Part model, mm, in its own coordinate system. A direction names the side the tool comes from. Give positions to 0.01 mm unless a question says otherwise; leave off trailing zeros. Write each loop counter-clockwise with the first axis right and the second up, starting at its lowest first coordinate (ties: lowest second). Pieces come first, ordered by that corner, then holes. Notation, with made-up numbers: M 83,-6 L 132,-6 A28 cw 132,19 Z; hole C -35,-8.5 d3. An arc over 180 degrees is marked long. Use CSV: the item, a comma, the result in double quotes. Start each with the question number.
1. 3-axis set-ups, long thin cutter, end or side, ignore diameter. For faces 1 (the face through (11, -7.62, 1)), 2 (the face through (3, -4, 22.86)), 3 (the face through (3, -5.08, 37)), 4 (the face through (8, -5, 20.32)), 5 (the face through (5.08, -8, 13)): which of +Z, -Z, +X, -X, +Y, -Y reach the whole face in a straight line?
2. Drill centre lines: line 1 along Z through (x, y) = (2, -3.25); line 2 along X through (y, z) = (-3, 12); line 3 along Y through (x, z) = (5, 20.5). Where is each one in solid material? Low to high. Write a range as from..to.
3. Band-saw the part on A-A, the plane y = -3. List the corners of the cut face in (x, z), then the cut area to 3 significant figures.
4. Band-saw the part on D-D, the plane y = -6. List the corners of the cut face in (x, z), then the cut area to 3 significant figures.
5. Mould opens along Z. For faces 6 (the face through (3, -4, 27.94)), 7 (the face through (7.62, -11, 1)), 8 (the face through (3, -3, 45.72)) say: pulls with the +Z half, pulls with the -Z half, needs draft (parallel to the pull), parting line crosses it, or undercut.
6. Drop flat-ended pins along their axis: pin 1 Ø5 at (y, z) = (-2.5, 8) entering from +X; pin 2 Ø0.8 at (x, y) = (2, -4) entering from -Z; pin 3 Ø2.5 at (x, z) = (3.5, 25.5) entering from -Y; pin 4 Ø0.8 at (x, z) = (11.5, 2) entering from +Y. Give the stop position or say it passes through.
7. Band-saw the part on B-B, the plane x = 4. List the corners of the cut face in (y, z).
8. Band-saw the part on C-C, the plane z = 24. List the corners of the cut face in (x, y), then the cut area to 3 significant figures.
from build123d import *

# Parameters (mm, degrees)
F0_W     = 10.16
F0_H     = 10.16
F1_DEPTH = 5.08
F2_W     = 5.08
F2_H     = 5.08
F3_DEPTH = 2.54
F4_W     = 5.08
F4_H     = 5.08
F5_DEPTH = 40.64
F6_W     = 5.08
F6_H     = 5.08
F7_DEPTH = 25.4
F8_W     = 5.08
F8_H     = 10.16
F9_DEPTH = 15.24


with BuildPart() as f1:
    # F0 (on Top) → F1 (new body)
    with BuildSketch(Plane.XY):
        with Locations((5.08, -5.08)):
            Rectangle(F0_W, F0_H)
    extrude(amount=F1_DEPTH)

    # F2 (on face) → F3 (join)
    with BuildSketch(Plane(origin=(0, 0, 0), x_dir=(1, 0, 0), z_dir=(0, 0, -1))):
        with Locations((10.16, 10.16)):
            Rectangle(F2_W, F2_H)
    extrude(amount=-F3_DEPTH)

    # F4 (on face) → F5 (join)
    with BuildSketch(Plane.XY.offset(5.08)):
        with Locations((2.54, -2.54)):
            Rectangle(F4_W, F4_H)
    extrude(amount=F5_DEPTH)

    # F6 (on face) → F7 (cut)
    with BuildSketch(Plane.YZ.offset(5.08)):
        with Locations((-5.08, 25.4)):
            Rectangle(F6_W, F6_H)
    extrude(amount=-F7_DEPTH, mode=Mode.SUBTRACT)

    # F8 (on face) → F9 (join)
    with BuildSketch(Plane.XY.offset(5.08)):
        with Locations((7.62, -5.08)):
            Rectangle(F8_W, F8_H)
    extrude(amount=F9_DEPTH)


solid = f1.part
Output:
1,face 1,"+Z, -Z, +X, +Y"
1,face 2,"+X, -X, -Y"
1,face 3,"+Z, +X, -X, -Y"
1,face 4,"+Z, +X, +Y, -Y"
1,face 5,"+Z, -X, -Y"
2,line 1,"z = 0..22.86, 27.94..45.72"
2,line 2,"x = 0..10.16"
2,line 3,"y = -5.08..0"
3,outline,"M 0,0 L 10.16,0 L 10.16,20.32 L 5.08,20.32 L 5.08,22.86 L 0,22.86 Z; M 0,27.94 L 5.08,27.94 L 5.08,45.72 L 0,45.72 Z"
3,area,"310 mm²"
4,outline,"M 0,0 L 10.16,0 L 10.16,20.32 L 5.08,20.32 L 5.08,5.08 L 0,5.08 Z"
4,area,"129 mm²"
5,face 6,"undercut"
5,face 7,"needs draft"
5,face 8,"pulls with the +Z half"
6,pin 1,"stops at x = 10.16"
6,pin 2,"stops at z = 0"
6,pin 3,"stops at y = -2.54"
6,pin 4,"stops at y = -7.62"
7,outline,"M -10.16,0 L 0,0 L 0,45.72 L -5.08,45.72 L -5.08,27.94 L -2.54,27.94 L -2.54,22.86 L -5.08,22.86 L -5.08,5.08 L -10.16,5.08 Z"
8,outline,"M 0,-2.54 L 5.08,-2.54 L 5.08,0 L 0,0 Z"
8,area,"12.9 mm²"
